For this review, take the finished solid that the model builds, in its own axes (mm). Give positions to 0.01 mm unless a question says otherwise; leave off trailing zeros. Order: outer loops, then holes, each group sorted by start corner. A loop starts at its lowest first (then second) coordinate and runs counter-clockwise, first axis right, second up.
Item 1: For P1, Ø1, axis at x = 16, y = 8.5, coming from the +Z side, flat-tipped, find the tip position at first contact; note if it passes through.
Item 2: Consider section A-A (z = 295.5). Give the boundary of the cut face in (x, y), plus the area to 3 significant figures.
Item 3: For probe 1 along Z at (x, y) = (0.95, 15); probe 2 along Y at (x, z) = (11.75, 98.5); probe 3 along X at (y, z) = (0.9, 384), list the stretches that pass through material, from the lowest coordinate up.
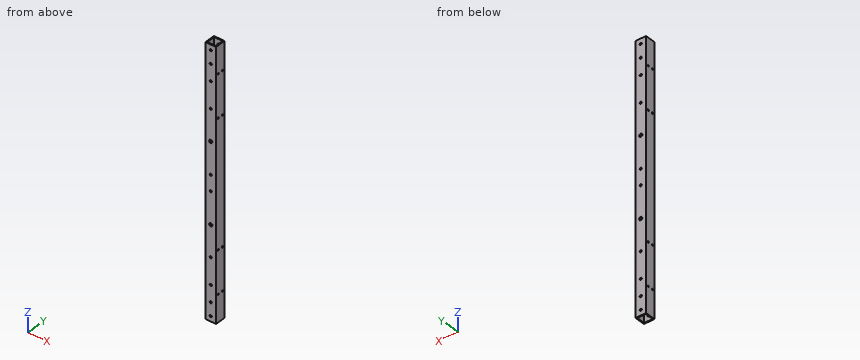
```python
from build123d import *

# Parameters (mm, degrees)
SKETCH_1_W          = 20
SKETCH_1_H          = 20
SKETCH_1_W_2        = 16
SKETCH_1_H_2        = 16
EXTRUDE_1_DEPTH     = 500
SKETCH_2_R          = 3
SKETCH_2_R_2        = 2
CUT_EXTRUDE_1_DEPTH = 501.799361022
SKETCH_3_R          = 1.5
CUT_EXTRUDE_2_DEPTH = 501.799361022
SKETCH_4_R          = 2
CUT_EXTRUDE_3_DEPTH = 501.799361022


with BuildPart() as part:
    # 草图1 → 凸台-拉伸1 (new body)
    with BuildSketch(Plane.XY):
        with Locations((10, 10)):
            Rectangle(SKETCH_1_W, SKETCH_1_H)
        with Locations((10, 10)):
            Rectangle(SKETCH_1_W_2, SKETCH_1_H_2, mode=Mode.SUBTRACT)
    extrude(amount=EXTRUDE_1_DEPTH)

    # 草图2 → 切除-拉伸1 (cut, through all)
    with BuildSketch(Plane(origin=(0, 0, 0), x_dir=(1, 0, 0), z_dir=(0, 1, 0))):
        with Locations(Location((10, -175, 0), (0, 0, 90))):
            Circle(SKETCH_2_R)
        with Locations(Location((10, -325, 0), (0, 0, 90))):
            Circle(SKETCH_2_R)
        with Locations(Location((10, -10, 0), (0, 0, 90))):
            Circle(SKETCH_2_R_2)
        with Locations(Location((10, -66, 0), (0, 0, 90))):
            Circle(SKETCH_2_R_2)
        with Locations(Location((10, -116, 0), (0, 0, 90))):
            Circle(SKETCH_2_R_2)
        with Locations(Location((10, -35, 0), (0, 0, 90))):
            Circle(SKETCH_2_R_2)
        with Locations(Location((10, -384, 0), (0, 0, 90))):
            Circle(SKETCH_2_R_2)
        with Locations(Location((10, -434, 0), (0, 0, 90))):
            Circle(SKETCH_2_R_2)
        with Locations(Location((10, -465, 0), (0, 0, 90))):
            Circle(SKETCH_2_R_2)
        with Locations(Location((10, -490, 0), (0, 0, 90))):
            Circle(SKETCH_2_R_2)
    extrude(amount=CUT_EXTRUDE_1_DEPTH, mode=Mode.SUBTRACT)

    # 草图3 → 切除-拉伸2 (cut, through all)
    with BuildSketch(Plane(origin=(0, 0, 0), x_dir=(0, 0, -1), z_dir=(1, 0, 0))):
        with Locations(Location((-449, 15, 0), (0, 0, 270))):
            Circle(SKETCH_3_R)
        with Locations(Location((-449, 5, 0), (0, 0, 180))):
            Circle(SKETCH_3_R)
        with Locations(Location((-369, 5, 0), (0, 0, 270))):
            Circle(SKETCH_3_R)
        with Locations(Location((-369, 15, 0), (0, 0, 180))):
            Circle(SKETCH_3_R)
        with Locations(Location((-131, 15, 0), (0, 0, 270))):
            Circle(SKETCH_3_R)
        with Locations(Location((-131, 5, 0), (0, 0, 180))):
            Circle(SKETCH_3_R)
        with Locations(Location((-51, 5, 0), (0, 0, 270))):
            Circle(SKETCH_3_R)
        with Locations(Location((-51, 15, 0), (0, 0, 180))):
            Circle(SKETCH_3_R)
    extrude(amount=CUT_EXTRUDE_2_DEPTH, mode=Mode.SUBTRACT)

    # 草图4 → 切除-拉伸3 (cut, through all)
    with BuildSketch(Plane(origin=(0, 20, 0), x_dir=(1, 0, 0), z_dir=(0, 1, 0))):
        with Locations(Location((10, -265, 0), (0, 0, 270))):
            Circle(SKETCH_4_R)
        with Locations(Location((10, -235, 0), (0, 0, 270))):
            Circle(SKETCH_4_R)
    extrude(amount=-CUT_EXTRUDE_3_DEPTH, mode=Mode.SUBTRACT)


solid = part.part
```
Resolved:
1. P1: passes through
2. outline: (0, 0) - (20, 0) - (20, 20) - (0, 20) - close; hole (2, 2) - (18, 2) - (18, 18) - (2, 18) - close
2. area: 144 mm2
3. probe 1: z = 0 to 49.5, 52.5 to 129.5, 132.5 to 367.5, 370.5 to 447.5, 450.5 to 500
3. probe 2: y = 0 to 2, 18 to 20
3. probe 3: x = 0 to 8, 12 to 20
